Work out the finished part from the listing and answer in its coordinate system (mm). A direction names the side the tool comes from. Give positions to 0.01 mm unless a question says otherwise; leave off trailing zeros. Loops run counter-clockwise (first coordinate to the right, second up) from the corner with the lowest first, then second, coordinate; pieces in that order, holes last. Notation, with made-up numbers: M -26,23 L 0,23 A26 ccw 0,57 Z; hole C -19,-2 d2. An arc over 180 degrees is marked long. Answer in a Markdown table with one row per item. Add a question column.
from build123d import *

# Parameters (mm, degrees)
SKETCH1_W           = 50
SKETCH1_H           = 50
BOSS_EXTRUDE1_DEPTH = 3.175
SKETCH2_W           = 3.175
SKETCH2_H           = 46.825
BOSS_EXTRUDE2_DEPTH = 14
SKETCH3_W           = 22
SKETCH3_H           = 8.1
SKETCH3_H_2         = 2.95
SKETCH3_R           = 0.5
CUT_EXTRUDE1_DEPTH  = 55.896089342
SKETCH4_W           = 22
SKETCH4_H           = 8.1
SKETCH4_H_2         = 2.95
SKETCH4_R           = 0.5
CUT_EXTRUDE2_DEPTH  = 55.896089342
SKETCH5_R           = 1.6
CUT_EXTRUDE3_DEPTH  = 40.306241553
FILLET1_R           = 1
FILLET2_R           = 15


with BuildPart() as part:
    # Sketch1 → Boss-Extrude1 (new body)
    with BuildSketch(Plane(origin=(0, 0, 0), x_dir=(1, 0, 0), z_dir=(0, 1, 0))):
        Rectangle(SKETCH1_W, SKETCH1_H)
    extrude(amount=BOSS_EXTRUDE1_DEPTH)

    # Sketch2 → Boss-Extrude2 (add)
    with BuildSketch(Plane(origin=(0, 0, 0), x_dir=(-1, 0, 0), z_dir=(0, -1, 0))):
        Polygon((-25, -25), (25, -25), (25, -21.825), (-21.825, -21.825), (-25, -21.825), align=None)
        with Locations((-23.4125, 1.5875)):
            Rectangle(SKETCH2_W, SKETCH2_H)
    extrude(amount=BOSS_EXTRUDE2_DEPTH)

    # Sketch3 → Cut-Extrude1 (cut, through all)
    with BuildSketch(Plane(origin=(0, 0, 21.825), x_dir=(-1, 0, 0), z_dir=(0, 0, -1))):
        with Locations((1.5875, -7)):
            Rectangle(SKETCH3_W, SKETCH3_H)
        with Locations((1.5875, -12.525)):
            Rectangle(SKETCH3_W, SKETCH3_H_2)
        with Locations((16.4475, -7)):
            Circle(SKETCH3_R)
    extrude(amount=-CUT_EXTRUDE1_DEPTH, mode=Mode.SUBTRACT)

    # Sketch4 → Cut-Extrude2 (cut, through all)
    with BuildSketch(Plane.ZY.offset(-21.825)):
        with Locations((-1.5875, -7)):
            Rectangle(SKETCH4_W, SKETCH4_H)
        with Locations((-1.5875, -12.525)):
            Rectangle(SKETCH4_W, SKETCH4_H_2)
        with Locations((13.2725, -7)):
            Circle(SKETCH4_R)
    extrude(amount=-CUT_EXTRUDE2_DEPTH, mode=Mode.SUBTRACT)

    # Sketch5 → Cut-Extrude3 (cut, through all)
    with BuildSketch(Plane(origin=(0, 3.175, 0), x_dir=(1, 0, 0), z_dir=(0, 1, 0))):
        with Locations(Location((-7.071067812, 17.928932188, 0), (0, 0, 270))):
            Circle(SKETCH5_R)
        with Locations(Location((-17.928932188, 7.071067812, 0), (0, 0, 270))):
            Circle(SKETCH5_R)
    extrude(amount=-CUT_EXTRUDE3_DEPTH, mode=Mode.SUBTRACT)

    # Fillet1
    fillet1_edges = [part.edges().sort_by_distance(p)[0] for p in [
        (-25, 3.175, 0),
        (0, 3.175, 25),
        (-1.5875, 0, -25),
        (-1.5875, 0, 21.825),
        (-25, -7, 21.825),
        (21.825, -14, -18.79375),
        (21.825, -7, -25),
        (-18.79375, -14, 21.825),
        (25, -14, -18.79375),
        (17.20625, -14, 25),
        (21.825, 0, -1.5875),
        (15.61875, -14, 21.825),
        (-18.79375, -14, 25),
        (25, 3.175, 0),
        (9.4125, -8.475, 21.825),
        (-1.5875, -2.95, 25),
        (-12.5875, -8.475, 25),
        (9.4125, -8.475, 25),
        (-12.5875, -8.475, 21.825),
        (-1.5875, -2.95, 21.825),
        (-25, 0, -1.5875),
        (21.825, -14, 15.61875),
        (25, -14, 17.20625),
        (21.825, -8.475, -12.5875),
        (25, -2.95, -1.5875),
        (25, -8.475, 9.4125),
        (23.4125, -14, 9.4125),
        (25, -8.475, -12.5875),
        (21.825, -8.475, 9.4125),
        (21.825, -2.95, -1.5875),
        (0, 3.175, -25),
        (25, -5.4125, 25),
        (-25, -5.4125, 25),
        (25, -5.4125, -25),
    ]]
    fillet(fillet1_edges, radius=FILLET1_R)

    # Fillet2
    # the kernel refuses this fillet: 15 mm, written as the material it takes off along each edge
    with BuildSketch(Plane(origin=(-10, 3.175, -10), x_dir=(0, 0, -1), z_dir=(1, 0, 0))) as fillet2_piece_1:
        with BuildLine():
            CenterArc((14, -1), 1, 0, 90)
            Line((15, -1), (15, 0))
            Line((15, 0), (14, 0))
        make_face()
    revolve(axis=Axis((-10, 3.175, -10), (0, 1, 0)), revolution_arc=90, mode=Mode.SUBTRACT)
    with BuildSketch(Plane(origin=(-10, 0, -10), x_dir=(-1, 0, 0), z_dir=(0, 0, 1))) as fillet2_piece_2:
        with BuildLine():
            CenterArc((14, -1), 1, 0, 90)
            Line((15, -1), (15, 0))
            Line((15, 0), (14, 0))
        make_face()
    revolve(axis=Axis((-10, 0, -10), (0, -1, 0)), revolution_arc=90, mode=Mode.SUBTRACT)
    with BuildSketch(Plane(origin=(-25, 0, -25), x_dir=(1, 0, 0), z_dir=(0, 1, 0))) as fillet2_piece_3:
        with BuildLine():
            CenterArc((FILLET2_R, -FILLET2_R), FILLET2_R, 90, 90)
            Line((0, -FILLET2_R), (0, 0))
            Line((0, 0), (FILLET2_R, 0))
        make_face()
    extrude(amount=3.175, mode=Mode.SUBTRACT)


solid = part.part
(1) Each of these flat-tipped pins is pushed along its axis until it touches: P1, Ø6, axis at x = 9, y = -10, coming from the -Z side (3 decimals); P2, Ø1.5, axis at y = -6.5, z = -13, coming from the +X side; P3, Ø0.9, axis at x = 23.5, z = 1, coming from the -Y side. Where does it stop, or does it pass through?
(2) Section B-B, the plane x = -0.5 is taken. Determine the outline of the cut face in (y, z) (3 decimals), and give its area (3 significant figures).
(3) Section C-C, the plane x = 15 is taken. Determine the outline of the cut face in (y, z) (3 decimals), and give its area (3 significant figures).
(4) Which of the six approach directions +Z, -Z, +X, -X, +Y, -Y give full straight-line access (tool end or side, diameter ignored) to faces 4 (the face through (-1.4, -1.6, 21.825)), 5 (the face through (23, -2.95, -2)), 6 (the face through (20, -14, 23)), 7 (the face through (-12.588, -9, 23))?
(5) Section A-A, the plane y = -4.25 is taken. Determine the outline of the cut face in (x, z) (1 decimal), and give its area (3 significant figures).
(6) The mould has two halves that part along Z. Classify faces 1 (the face through (12.1, 1.3, -25)), 2 (the face through (-8.04, 1.61, -19.2)), 3 (the face through (-1, -2.95, 23)): pulls with the +Z half, pulls with the -Z half, needs draft (parallel to the pull), parting line crosses it, or undercut.
(7) Consider line 1 along X through (y, z) = (-10.25, -22) (3 decimals); line 2 along X through (y, z) = (-7.75, 23.5); line 3 along Y through (x, z) = (-7, -15.5) (3 decimals). Determine where each line is inside the solid, lowest interval first. Write a range as from..to.
Numbers:
| question | item | result |
|---|---|---|
| 1 | P1 | stops at z = 21.825 |
| 1 | P2 | stops at x = 25 |
| 1 | P3 | stops at y = -2.95 |
| 2 | outline | M -2.95,22.825 A1 ccw -1.95,21.825 L -1,21.825 A1 cw 0,20.825 L 0,-24 A1 ccw 1,-25 L 2.175,-25 A1 ccw 3.175,-24 L 3.175,24 A1 ccw 2.175,25 L -1.95,25 A1 ccw -2.95,24 Z |
| 2 | area | 167 mm² |
| 3 | outline | M -14,22.825 A1 ccw -13,21.825 L -1,21.825 A1 cw 0,20.825 L 0,-24 A1 ccw 1,-25 L 2.175,-25 A1 ccw 3.175,-24 L 3.175,24 A1 ccw 2.175,25 L -13,25 A1 ccw -14,24 Z |
| 3 | area | 202 mm² |
| 4 | face 4 | -Z, -X, -Y |
| 4 | face 5 | +X, -X, -Y |
| 4 | face 6 | +Z, -Z, +X, -X, -Y |
| 4 | face 7 | +Z, -Z, -Y |
| 5 | outline | M -25,22.8 A1 ccw -24,21.8 L -13.6,21.8 A1 ccw -12.6,22.8 L -12.6,24 A1 ccw -13.6,25 L -24,25 A1 ccw -25,24 Z; M 9.4,22.8 A1 ccw 10.4,21.8 L 21.8,21.8 L 21.8,10.4 A1 ccw 22.8,9.4 L 24,9.4 A1 ccw 25,10.4 L 25,24 A1 ccw 24,25 L 10.4,25 A1 ccw 9.4,24 Z; M 21.8,-24 A1 ccw 22.8,-25 L 24,-25 A1 ccw 25,-24 L 25,-13.6 A1 ccw 24,-12.6 L 22.8,-12.6 A1 ccw 21.8,-13.6 Z |
| 5 | area | 165 mm² |
| 6 | face 1 | pulls with the -Z half |
| 6 | face 2 | undercut |
| 6 | face 3 | needs draft |
| 7 | line 1 | x = 21.825..25 |
| 7 | line 2 | x = -25..-12.59, 9.41..25 |
| 7 | line 3 | y = 0..3.175 |
